The listing builds one solid part. Answer for the finished solid, in the listing's coordinates (mm). A direction names the side the tool comes from. Give positions to 0.01 mm unless a question says otherwise; leave off trailing zeros. Order: outer loops, then holes, each group sorted by start corner. A loop starts at its lowest first (then second) coordinate and runs counter-clockwise, first axis right, second up. Notation, with made-up numbers: (44, -9.75) - (76, -9.75) arc R10 cw to (76, 8.25) - close; hole circle Ø6 at (9, 36.25). An arc over 180 degrees is marked (long way). Answer as a JSON object with one key per item and string values. Group by question number.
Q1. A cutting plane is placed at D-D, the plane z = -8. Give the vertices of the cut face in (x, y).
Q2. Given pin 1 (6 mm diameter, centred on y = 48, z = -37.5, fed in from +X); pin 2 (15 mm diameter, centred on x = 30.5, z = -24.5, fed in from +Y); pin 3 (21.5 mm diameter, centred on y = 25, z = -25, fed in from -X); pin 4 (1.5 mm diameter, centred on x = 15.5, z = -15.5, fed in from +Y), each flat-ended and moving along its own axis, determine where each tip first touches the part or whether it passes through.
Q3. A cutting plane is placed at B-B, the plane x = 25. Give the vertices of the cut face in (y, z).
Q4. Consider line 1 (X direction, y = 3, z = -25); line 2 (Y direction, x = 38, z = -19.5). Determine where each line is inside the solid, lowest interval first.
Q5. For faces 1 (the face through (52.465, 37.203, -27.71)), 2 (the face through (32.606, 52.465, -15.08)), 3 (the face through (19.83, 2.46, -37.47)), 4 (the face through (25, 25, -45)), 5 (the face through (2.46, 19.83, -12.53)), determine the directions among +Z, -Z, +X, -X, +Y, -Y from which every point of the face is accessible in a straight line to the end or side of a thin tool.
Q6. The mould has two halves that part along Y. Classify faces 6 (the face through (0, 36, -36)), 7 (the face through (20, 5, -12)), 8 (the face through (30, 55, -36)): released by +Y, released by -Y, zero draft, split by the parting line, or undercut.
Q7. A cutting plane is placed at A-A, the plane z = -25. Count the separate pieces of the cut face and the enclosed holes in it, and give its area (3 significant figures).
from build123d import *

# Parameters (mm, degrees)
SKETCH1_W           = 50
SKETCH1_H           = 50
BOSS_EXTRUDE1_DEPTH = 50
SKETCH2_W           = 40
SKETCH2_H           = 40
CUT_EXTRUDE1_DEPTH  = 45
SKETCH3_R           = 12.5
BOSS_EXTRUDE2_DEPTH = 5
SKETCH4_R           = 13.5
CUT_EXTRUDE2_DEPTH  = 5
SKETCH5_R           = 12.5
BOSS_EXTRUDE3_DEPTH = 5
SKETCH6_R           = 13.5
CUT_EXTRUDE3_DEPTH  = 5
SKETCH7_R           = 11.75
CUT_EXTRUDE4_DEPTH  = 10
SKETCH8_R           = 11.75
CUT_EXTRUDE5_DEPTH  = 10


with BuildPart() as part:
    # Sketch1 → Boss-Extrude1 (new body)
    with BuildSketch(Plane(origin=(0, 0, 0), x_dir=(1, 0, 0), z_dir=(0, 1, 0))):
        with Locations((25, 25)):
            Rectangle(SKETCH1_W, SKETCH1_H)
    extrude(amount=BOSS_EXTRUDE1_DEPTH)

    # Sketch2 → Cut-Extrude1 (cut)
    with BuildSketch(Plane.XY):
        with Locations((25, 25)):
            Rectangle(SKETCH2_W, SKETCH2_H)
    extrude(amount=-CUT_EXTRUDE1_DEPTH, mode=Mode.SUBTRACT)

    # Sketch3 → Boss-Extrude2 (add)
    with BuildSketch(Plane(origin=(0, 50, 0), x_dir=(1, 0, 0), z_dir=(0, 1, 0))):
        with Locations(Location((25, 25, 0), (0, 0, 90))):
            Circle(SKETCH3_R)
    extrude(amount=BOSS_EXTRUDE2_DEPTH)

    # Sketch4 → Cut-Extrude2 (cut)
    with BuildSketch(Plane.XZ):
        with Locations(Location((25, -25, 0), (0, 0, 270))):
            Circle(SKETCH4_R)
    extrude(amount=-CUT_EXTRUDE2_DEPTH, mode=Mode.SUBTRACT)

    # Sketch5 → Boss-Extrude3 (add)
    with BuildSketch(Plane(origin=(50, 0, 0), x_dir=(0, 0, -1), z_dir=(1, 0, 0))):
        with Locations(Location((25, 25, 0), (0, 0, 180))):
            Circle(SKETCH5_R)
    extrude(amount=BOSS_EXTRUDE3_DEPTH)

    # Sketch6 → Cut-Extrude3 (cut)
    with BuildSketch(Plane.ZY):
        with Locations((-25, 25)):
            Circle(SKETCH6_R)
    extrude(amount=-CUT_EXTRUDE3_DEPTH, mode=Mode.SUBTRACT)

    # Sketch7 → Cut-Extrude4 (cut)
    with BuildSketch(Plane(origin=(0, 55, 0), x_dir=(1, 0, 0), z_dir=(0, 1, 0))):
        with Locations(Location((25, 25, 0), (0, 0, 270))):
            Circle(SKETCH7_R)
    extrude(amount=-CUT_EXTRUDE4_DEPTH, mode=Mode.SUBTRACT)

    # Sketch8 → Cut-Extrude5 (cut)
    with BuildSketch(Plane(origin=(55, 0, 0), x_dir=(0, 0, -1), z_dir=(1, 0, 0))):
        with Locations((25, 25)):
            Circle(SKETCH8_R)
    extrude(amount=-CUT_EXTRUDE5_DEPTH, mode=Mode.SUBTRACT)


solid = part.part
Reply:
{
 "1": {"outline": "(0, 0) - (50, 0) - (50, 50) - (0, 50) - close; hole (5, 5) - (45, 5) - (45, 45) - (5, 45) - close"},
 "2": {"pin 1": "stops at x = 50", "pin 2": "stops at y = 55", "pin 3": "passes through", "pin 4": "stops at y = 50"},
 "3": {"outline": "(0, -50) - (50, -50) - (50, -37.5) - (55, -37.5) - (55, -36.75) - (45, -36.75) - (45, -45) - (5, -45) - (5, -38.5) - (0, -38.5) - close; (0, -11.5) - (5, -11.5) - (5, 0) - (0, 0) - close; (45, -13.25) - (55, -13.25) - (55, -12.5) - (50, -12.5) - (50, 0) - (45, 0) - close"},
 "4": {"line 1": "x = 0 to 11.5, 38.5 to 50", "line 2": "y = 0 to 5, 45 to 50"},
 "5": {"face 1": "+X", "face 2": "+Y", "face 3": "-Y", "face 4": "+Z", "face 5": "-X"},
 "6": {"face 6": "zero draft", "face 7": "undercut", "face 8": "released by +Y"},
 "7": {"separate pieces": "4", "enclosed holes": "0", "area": "410 mm^2"}
}
